Verification items for the finished model (mm, model axes). Face numbers are marked on the shaded views. Coordinates: 2 decimals unless noted, no trailing zeros. Order: outer loops, then holes, each group sorted by start corner. A loop starts at its lowest first (then second) coordinate and runs counter-clockwise, first axis right, second up. Notation, with made-up numbers: (40.25, 22.5) -> (57.25, 22.5) arc R29 ccw to (57.25, 57.5) -> close; hole circle Ø5 at (9.5, 45). An arc over 180 degrees is marked (long way). Write item = value, one per line. Start each with the question number.
1. Go/stop test with flat-tipped pins: P1, Ø1.5, axis at x = -0.5, y = -15, coming from the +Z side; P2, Ø3, axis at x = -23.5, y = 9, coming from the -Z side. Record where each tip stops, or that it passes through.
2. Release check for a two-part mould opening along Y. For the marked faces 1, 2, 3 and 4 record: +Y half, -Y half, draft (parallel to the pull), parting line (faces both ways), or undercut.
3. Thickness scan on line 1 along X through (y, z) = (1, 2.4); line 2 along Y through (x, z) = (-13.5, 2.9). Record the ranges inside material, lowest first. Write a range as from..to.
4. Cross-section at A-A on z = 2.2. Record the cut outline in (x, y), plus the area to 3 significant figures.
5. Cross-section at C-C on x = 0. Record the cut outline in (y, z).
6. Cross-section at B-B on y = -7. Record the cut outline in (x, z), plus the area to 3 significant figures.
from build123d import *

# Parameters (mm, degrees)
F0_W     = 60
F0_H     = 60
F1_DEPTH = 5
F2_R     = 25
F3_DEPTH = 2
F4_R     = 10
F5_W     = 6
F5_H     = 3
F5_W_2   = 3
F5_H_2   = 6
F6_DEPTH = 2


with BuildPart() as f1:
    # F0 (on Top) → F1 (new body)
    with BuildSketch(Plane.XY):
        Rectangle(F0_W, F0_H)
    extrude(amount=F1_DEPTH)

    # F2 (on face) → F3 (cut)
    with BuildSketch(Plane.XY.offset(5)):
        Circle(F2_R)
    extrude(amount=-F3_DEPTH, mode=Mode.SUBTRACT)

    # F4
    f4_edges = [f1.edges().sort_by_distance(p)[0] for p in [
        (30, -30, 2.5),
        (30, 30, 2.5),
        (-30, 30, 2.5),
        (-30, -30, 2.5),
    ]]
    fillet(f4_edges, radius=F4_R)

    # F5 (on face) → F6 (cut)
    with BuildSketch(Plane.XY.offset(3)):
        with Locations((-16, 0)):
            Rectangle(F5_W, F5_H)
        with Locations((0, 16)):
            Rectangle(F5_W_2, F5_H_2)
        with Locations((16, 0)):
            Rectangle(F5_W, F5_H)
        with Locations((0, -16)):
            Rectangle(F5_W_2, F5_H_2)
    extrude(amount=-F6_DEPTH, mode=Mode.SUBTRACT)


solid = f1.part
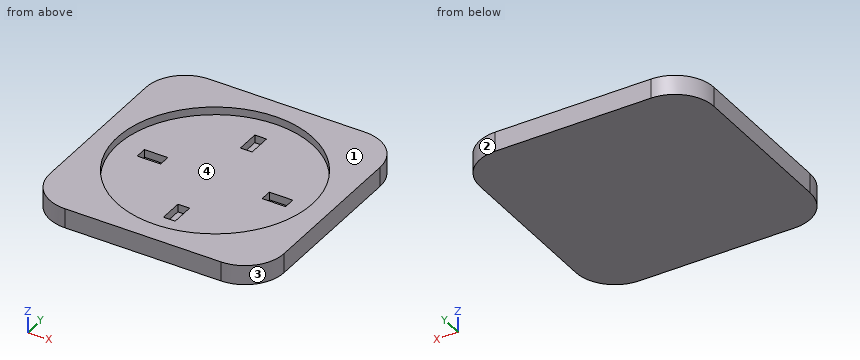
Worked out:
q1.P1 = 1
q1.P2 = 0
q2.face_1 = draft
q2.face_2 = +Y half
q2.face_3 = -Y half
q2.face_4 = undercut
q3.line_1 = -30..-19, -13..13, 19..30
q3.line_2 = -30..-1.5, 1.5..30
q4.outline = (-30, -20) arc R10 ccw to (-20, -30) -> (20, -30) arc R10 ccw to (30, -20) -> (30, 20) arc R10 ccw to (20, 30) -> (-20, 30) arc R10 ccw to (-30, 20) -> close; hole (-19, -1.5) -> (-13, -1.5) -> (-13, 1.5) -> (-19, 1.5) -> close; hole (-1.5, -19) -> (1.5, -19) -> (1.5, -13) -> (-1.5, -13) -> close; hole (-1.5, 13) -> (1.5, 13) -> (1.5, 19) -> (-1.5, 19) -> close; hole (13, -1.5) -> (19, -1.5) -> (19, 1.5) -> (13, 1.5) -> close
q4.area = 3,440 mm²
q5.outline = (-30, 0) -> (30, 0) -> (30, 5) -> (25, 5) -> (25, 3) -> (19, 3) -> (19, 1) -> (13, 1) -> (13, 3) -> (-13, 3) -> (-13, 1) -> (-19, 1) -> (-19, 3) -> (-25, 3) -> (-25, 5) -> (-30, 5) -> close
q6.outline = (-30, 0) -> (30, 0) -> (30, 5) -> (24, 5) -> (24, 3) -> (-24, 3) -> (-24, 5) -> (-30, 5) -> close
q6.area = 204 mm²
